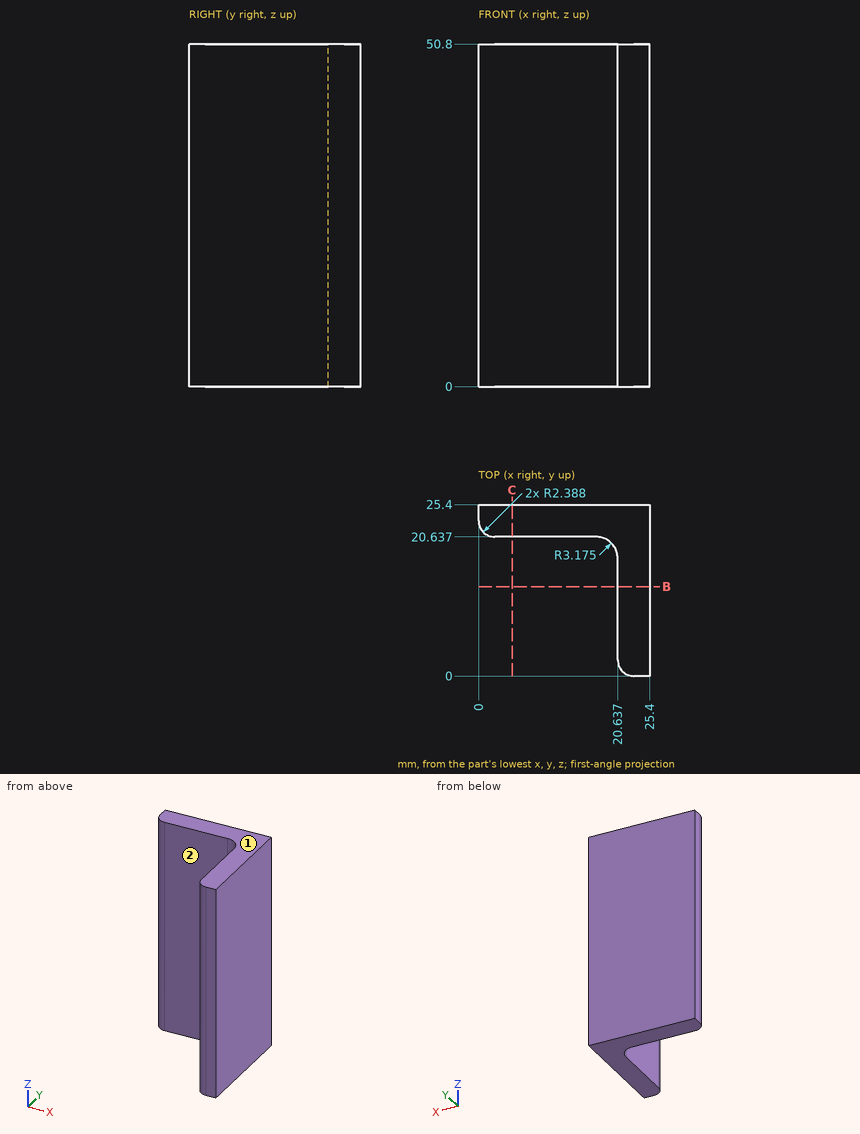
Could you check a few things on this drawing? It's one solid part, dimensions in mm from its lowest x, y, z. A direction names the side the tool comes from. Round coordinates to 2 decimals unless told otherwise and drop trailing zeros. Loops run counter-clockwise (first coordinate to the right, second up) from the corner with the lowest first, then second, coordinate; pieces in that order, holes last. Notation, with made-up numbers: M -5.5,-14 L 48.5,-14 A26 cw 48.5,6 Z; hole C 31.25,61.25 d4. An arc over 180 degrees is marked long. Write item = value, one per line. Start each with the question number.
(1) Suppose I cut it at B-B on y = 13.25. Write out the boundary of the cut face in (x, z), plus the area to 3 significant figures.
(2) Which directions (+Z, -Z, +X, -X, +Y, -Y) give clear straight access to the entire face, cutting with the end or side of a thin tool? Please do the marked faces 1 and 2.
(3) I'm going to push flat-ended pins straight in: P1, Ø8, axis at y = 3, z = 45.5, coming from the -X side; P2, Ø4.5, axis at x = 12, z = 23, coming from the -Y side. Where does each tip first touch, or does it pass through?
(4) I need wall thicknesses on line 1 along X through (y, z) = (11.75, 8.5); line 2 along X through (y, z) = (21.5, 47). Which ranges of each line are inside material? Lowest first, please.
Answer block:
q1.outline = M 20.64,0 L 25.4,0 L 25.4,50.8 L 20.64,50.8 Z
q1.area = 242 mm²
q2.face_1 = +Z, +X, -X, +Y, -Y
q2.face_2 = +Z, -Z, -X, -Y
q3.P1 = 20.64
q3.P2 = 20.64
q4.line_1 = 20.64 to 25.4
q4.line_2 = 0.55 to 25.4
